Autodesk Inventor part; units mm, degrees
ref_plane "YZ Plane" through (0, 0, 0) normal (1, 0, 0) x (0, 1, 0)
ref_plane "XZ Plane" through (0, 0, 0) normal (0, 1, 0) x (-1, 0, 0)
ref_plane "XY Plane" through (0, 0, 0) normal (0, 0, 1) x (1, 0, 0)
sketch "Sketch1" plane through (0, 0, 0) normal (0, 1, 0) x (-1, 0, 0)
  line L0 (0, 0) -> (284.48, 0)
  line L1 (284.48, 0) -> (284.48, 111.76)
  line L2 (284.48, 111.76) -> (0, 111.76)
  line L3 (0, 111.76) -> (0, 0)
  dimension "d0" = 284.48
  dimension "d1" = 111.76
extrude "Extrusion1" add sketch "Sketch1" along normal blind 20.32
sketch "Sketch2" plane through (0, 20.32, 0) normal (0, 1, 0) x (1, 0, 0)
  line L0 (-284.48, 0) -> (-284.48, -111.76)
  line L1 (0, -111.76) -> (0, 0)
  line L2 (-284.48, -55.88) -> (-257.175, -55.88) construction
  line L3 (0, -55.88) -> (-27.305, -55.88) construction
  circle A0 centre (-27.305, -55.88) radius 12.7
  circle A1 centre (-257.175, -55.88) radius 12.7
  dimension "d4" = 27.305
  dimension "d5" = 27.305
  dimension "d6" = 25.4
  dimension "d7" = 25.4
extrude "Extrusion2" cut sketch "Sketch2" against normal blind 20.32
fillet "Fillet1" radius 4 4 edges at (-284.48, 10.16, 111.76) (-284.48, 10.16, 0) (0, 10.16, 111.76) (0, 10.16, 0)
fillet "Fillet2" radius 1 16 edges at (-283.3084, 0, 1.1716) (-284.48, 0, 55.88) (-283.3084, 0, 110.5884) (-142.24, 0, 111.76) (-1.1716, 0, 110.5884) (0, 0, 55.88) (-1.1716, 0, 1.1716) (-142.24, 0, 0) (-283.3084, 20.32, 1.1716) (-284.48, 20.32, 55.88) (-283.3084, 20.32, 110.5884) (-142.24, 20.32, 111.76) (-1.1716, 20.32, 110.5884) (0, 20.32, 55.88) (-1.1716, 20.32, 1.1716) (-142.24, 20.32, 0)
equation "\"d5\" = d4"
properties part number "CIM Mount Top" material "Aluminum 6061"
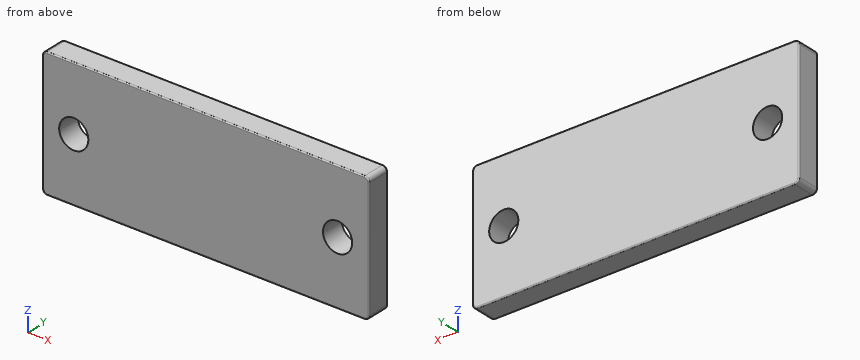
Geometry: final body of the model. Coordinates: model frame, mm. Coordinates: 2 decimals unless noted, no trailing zeros. Order: outer loops, then holes, each group sorted by start corner. A loop starts at its lowest first (then second) coordinate and runs counter-clockwise, first axis right, second up. Notation, with made-up numbers: M -23.75,-28.5 L 2.25,-28.5 A7 ccw 2.25,-24.5 Z; hole C 43,69 d11. An arc over 180 degrees is marked long. Answer in a Markdown table with one row per item. Add a question column.
Q1. Line query: L1, parallel to X at y = 14.25, z = 55.88 (3 decimals); L2, parallel to X at y = 8.25, z = 45.5; L3, parallel to Z at x = -36, y = 5.25. Output: solid intervals per line, ascending.
Q2. Section query A-A on z = 55.88. Return the cut outline in (x, y) (3 decimals).
Q3. Section query B-B on y = 9. Return the cut outline in (x, z) (3 decimals), and give its area (3 significant figures).
Completed:
| question | item | result |
|---|---|---|
| 1 | L1 | x = -284.48 to -269.875, -244.475 to -40.005, -14.605 to 0 |
| 1 | L2 | x = -284.48 to -264.49, -249.86 to -34.62, -19.99 to 0 |
| 1 | L3 | z = 0 to 46.62, 65.14 to 111.76 |
| 2 | outline | M -284.48,1 A1 ccw -283.48,0 L -269.875,0 L -269.875,20.32 L -283.48,20.32 A1 ccw -284.48,19.32 Z; M -244.475,0 L -40.005,0 L -40.005,20.32 L -244.475,20.32 Z; M -14.605,0 L -1,0 A1 ccw 0,1 L 0,19.32 A1 ccw -1,20.32 L -14.605,20.32 Z |
| 3 | outline | M -284.48,4 A4 ccw -280.48,0 L -4,0 A4 ccw 0,4 L 0,107.76 A4 ccw -4,111.76 L -280.48,111.76 A4 ccw -284.48,107.76 Z; hole C -257.175,55.88 d25.4; hole C -27.305,55.88 d25.4 |
| 3 | area | 30,800 mm2 |
